Can you work these out from the model? Positions are in its coordinate system, mm. A direction names the side the tool comes from. Coordinates: 2 decimals unless noted, no trailing zeros. Order: outer loops, then holes, each group sorted by start corner. A loop starts at its lowest first (then second) coordinate and runs counter-clockwise, first axis right, second up. Notation, with made-up numbers: (48.25, 89.25) -> (82.25, 89.25) arc R31 ccw to (82.25, 113.25) -> close; hole circle Ø8 at (4.5, 1.5). An arc over 180 degrees is marked (long way). Answer in a Markdown table with one row per item. Add a question column.
1. Imagine slicing it at B-B on y = -68. Write out the boundary of the cut face in (x, z).
2. Imagine slicing it at C-C on x = -41. Write out the boundary of the cut face in (y, z), plus the area to 3 significant figures.
3. Imagine slicing it at A-A on z = 79.5. Write out the boundary of the cut face in (x, y), plus the area to 3 significant figures.
4. Will these pins go through, and if not, where does the flat tip stop? pin 1 (2 mm diameter, centred on x = -24, y = 61, fed in from -Z); pin 2 (5 mm diameter, centred on x = -11, y = -34.5, fed in from +Z).
5. We'd pull the mould along Y, two halves only. Please class faces 1 (the face through (-48.297, -2, 52)), 2 (the face through (-22.505, -116.315, 97.535)), 3 (the face through (11.968, -2, 47)): pulls with the +Y half, pulls with the -Y half, needs draft (parallel to the pull), parting line crosses it, or undercut.
6. If I drill on line 1 along X through (y, z) = (38.5, 73.5); line 2 along Y through (x, z) = (1, 9.5); line 3 along Z through (x, y) = (-43, 27), over which ranges is the centre line in solid material (lowest first)? Write a range as [from, to].
7. On a 3-axis mill with a long thin cutter (end or side, diameter ignored), from which of +Z, -Z, +X, -X, +Y, -Y can I reach the whole of each face in a straight line? I mean faces 4 (the face through (-22, -2, 5)), 5 (the face through (-22, 118.85, 47)). Say none if no direction works.
from build123d import *

# Parameters (mm, degrees)
F0_W     = 68.029277
F0_H     = 237.70012
F0_W_2   = 52.5
F0_H_2   = 225
F1_DEPTH = 100
F2_W     = 225
F2_H     = 5
F3_DEPTH = 52.5
F4_SIZE  = 5
F5_SIZE  = 2.5


with BuildPart() as f1:
    # F0 (on Top) → F1 (new body)
    with BuildSketch(Plane.XY):
        with Locations((-22.046504, 0)):
            Rectangle(F0_W, F0_H)
        with Locations((-22.046504, 0)):
            Rectangle(F0_W_2, F0_H_2, mode=Mode.SUBTRACT)
    extrude(amount=F1_DEPTH)

    # F2 (on face) → F3 (join)
    with BuildSketch(Plane.YZ.offset(-48.296504)):
        with Locations((0, 2.5)):
            Rectangle(F2_W, F2_H)
    extrude(amount=F3_DEPTH)

    # F4
    f4_edges = [f1.edges().sort_by_distance(p)[0] for p in [
        (-56.061142, 0, 100),
        (-22.046504, -118.85006, 100),
        (11.968135, 0, 100),
        (-22.046504, 118.85006, 100),
    ]]
    chamfer(f4_edges, length=F4_SIZE)

    # F5
    f5_edges = [f1.edges().sort_by_distance(p)[0] for p in [
        (-56.061142, -118.85006, 47.5),
        (11.968135, -118.85006, 47.5),
        (11.968135, 118.85006, 47.5),
        (-56.061142, 118.85006, 47.5),
    ]]
    chamfer(f5_edges, length=F5_SIZE)


solid = f1.part
Answers follow:
| question | item | result |
|---|---|---|
| 1 | outline | (-56.06, 0) -> (11.97, 0) -> (11.97, 95) -> (6.97, 100) -> (4.2, 100) -> (4.2, 5) -> (-48.3, 5) -> (-48.3, 100) -> (-51.06, 100) -> (-56.06, 95) -> close |
| 2 | outline | (-118.85, 0) -> (118.85, 0) -> (118.85, 95) -> (113.85, 100) -> (112.5, 100) -> (112.5, 5) -> (-112.5, 5) -> (-112.5, 100) -> (-113.85, 100) -> (-118.85, 95) -> close |
| 2 | area | 2,370 mm² |
| 3 | outline | (-56.06, -116.35) -> (-53.56, -118.85) -> (9.47, -118.85) -> (11.97, -116.35) -> (11.97, 116.35) -> (9.47, 118.85) -> (-53.56, 118.85) -> (-56.06, 116.35) -> close; hole (-48.3, -112.5) -> (4.2, -112.5) -> (4.2, 112.5) -> (-48.3, 112.5) -> close |
| 3 | area | 4,350 mm² |
| 4 | pin 1 | stops at z = 0 |
| 4 | pin 2 | stops at z = 5 |
| 5 | face 1 | undercut |
| 5 | face 2 | pulls with the -Y half |
| 5 | face 3 | needs draft |
| 6 | line 1 | x = [-56.06, -48.3], [4.2, 11.97] |
| 6 | line 2 | y = [-118.85, -112.5], [112.5, 118.85] |
| 6 | line 3 | z = [0, 5] |
| 7 | face 4 | +Z |
| 7 | face 5 | +Z, -Z, +X, -X, +Y |
